```python
from build123d import *

# Parameters (mm, degrees)
SKETCH_1_R          = 3
EXTRUDE_1_DEPTH     = 6
SKETCH_2_R          = 3.1
CUT_EXTRUDE_6_DEPTH = 3
SKETCH_4_R          = 1.5
CUT_EXTRUDE_7_DEPTH = 129.481995307


with BuildPart() as part:
    # 草图1 → 凸台-拉伸1 (new body)
    with BuildSketch(Plane.XY):
        with BuildLine():
            Line((55.4927663, 10.009964479), (83.62403307, -87.496893342))
            Line((83.62403307, -87.496893342), (83.62403307, -97.496893342))
            Line((83.62403307, -97.496893342), (-16.37596693, -97.496893342))
            Line((-16.37596693, -97.496893342), (-16.37596693, -87.496893342))
            Line((-16.37596693, -87.496893342), (17.356392529, 10.94893296))
            ThreePointArc((17.356392529, 10.94893296), (36.768797098, 24.459911865), (55.4927663, 10.009964479))
        make_face()
        with Locations((36.276519563, 4.465971212)):
            Circle(SKETCH_1_R, mode=Mode.SUBTRACT)
    extrude(amount=EXTRUDE_1_DEPTH)

    # 草图2 → 切除-拉伸6 (cut)
    with BuildSketch(Plane.XY.offset(6)):
        with Locations((29.276519563, 11.465971212)):
            Circle(SKETCH_2_R)
        with Locations(Location((43.276519563, 11.465971212, 0), (0, 0, 180))):
            Circle(SKETCH_2_R)
        with Locations((43.276519563, -2.534028788)):
            Circle(SKETCH_2_R)
        with Locations(Location((29.276519563, -2.534028788, 0), (0, 0, 180))):
            Circle(SKETCH_2_R)
    extrude(amount=-CUT_EXTRUDE_6_DEPTH, mode=Mode.SUBTRACT)

    # 草图4 → 切除-拉伸7 (cut, through all)
    with BuildSketch(Plane.XY.offset(3)):
        with Locations((43.276519563, 11.465971212)):
            Circle(SKETCH_4_R)
        with Locations((43.276519563, -2.534028788)):
            Circle(SKETCH_4_R)
        with Locations((29.276519563, -2.534028788)):
            Circle(SKETCH_4_R)
        with Locations((29.276519563, 11.465971212)):
            Circle(SKETCH_4_R)
    extrude(amount=-CUT_EXTRUDE_7_DEPTH, mode=Mode.SUBTRACT)


solid = part.part
```
Here's how the part is built. I have some questions about the finished solid (model axes, mm). A direction names the side the tool comes from. Coordinates: 2 decimals unless noted, no trailing zeros. Order: outer loops, then holes, each group sorted by start corner. A loop starts at its lowest first (then second) coordinate and runs counter-clockwise, first axis right, second up.
1) We'd pull the mould along Y, two halves only. Please class faces 1 (the face through (-16.376, -93, 3)), 2 (the face through (33.28, 4.6, 2.96)), 3 (the face through (69.36, -38.06, 2.96)): +Y half, -Y half, draft (parallel to the pull), parting line (faces both ways), or undercut.
2) Imagine slicing it at C-C on y = -66. List the corners of the cut face in (x, z) for me.
3) Imagine slicing it at A-A on x = 43.5. List the corners of the cut face in (y, z) for me.
4) Which directions (+Z, -Z, +X, -X, +Y, -Y) give clear straight access to the entire face, cutting with the end or side of a thin tool? Please do faces 4 (the face through (36.415, 24.465, 2.958)), 5 (the face through (31, 12, 3)).
5) Will these pins go through, and if not, where does the flat tip stop? pin 1 (1 mm diameter, centred on y = -6.5, z = 4.5, fed in from -X); pin 2 (1.9 mm diameter, centred on x = 28.5, y = -2.5, fed in from +Z); pin 3 (2 mm diameter, centred on x = 52.5, z = 4.5, fed in from +Y).
6) Imagine slicing it at B-B on z = 2.1. List the corners of the cut face in (x, y) for me.
7) I need wall thicknesses on line 1 (Y direction, x = 42.5, z = 2.8); line 2 (Y direction, x = 43, z = 3.7); line 3 (X direction, y = -5, z = 4.4). Which ranges of each line are inside material? Lowest first, please.
8) Imagine slicing it at D-D on x = 24. List the corners of the cut face in (y, z) for me.
Response values:
1. face 1: draft
1. face 2: undercut
1. face 3: +Y half
2. outline: (-9.01, 0) - (77.42, 0) - (77.42, 6) - (-9.01, 6) - close
3. outline: (-97.5, 0) - (-4.02, 0) - (-4.02, 3) - (-5.63, 3) - (-5.63, 6) - (-97.5, 6) - close; (-1.05, 0) - (9.98, 0) - (9.98, 3) - (8.37, 3) - (8.37, 6) - (0.56, 6) - (0.56, 3) - (-1.05, 3) - close; (12.95, 0) - (23.12, 0) - (23.12, 6) - (14.56, 6) - (14.56, 3) - (12.95, 3) - close
4. face 4: +Z, -Z, +Y
4. face 5: +Z
5. pin 1: stops at x = 11.21
5. pin 2: stops at z = 3
5. pin 3: stops at y = 17.44
6. outline: (-16.38, -97.5) - (83.62, -97.5) - (83.62, -87.5) - (55.49, 10.01) arc R20 ccw to (17.36, 10.95) - (-16.38, -87.5) - close; hole circle Ø3 at (29.28, -2.53); hole circle Ø3 at (29.28, 11.47); hole circle Ø6 at (36.28, 4.47); hole circle Ø3 at (43.28, -2.53); hole circle Ø3 at (43.28, 11.47)
7. line 1: y = -97.5 to -3.82, -1.25 to 10.18, 12.75 to 23.47
7. line 2: y = -97.5 to -5.62, 0.55 to 8.38, 14.55 to 23.3
7. line 3: x = 11.89 to 27.4, 31.16 to 41.4, 45.16 to 59.82
8. outline: (-97.5, 0) - (20.25, 0) - (20.25, 6) - (-97.5, 6) - close
